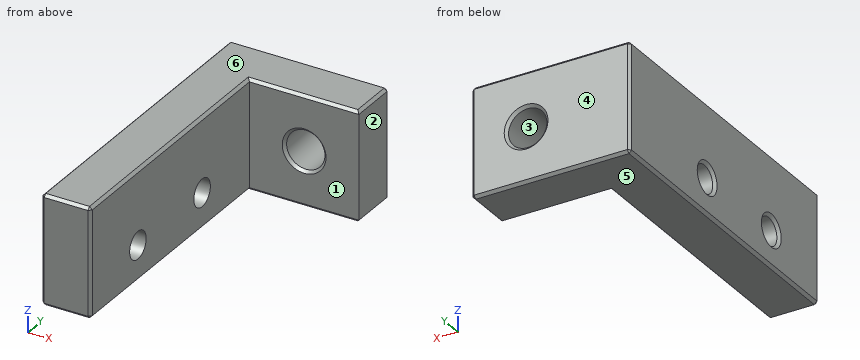
```python
from build123d import *

# Parameters (mm, degrees)
BOSS_EXTRUDE1_DEPTH = 10
SKETCH2_R           = 1.75
CUT_EXTRUDE1_DEPTH  = 10
SKETCH3_R           = 1.25
CUT_EXTRUDE2_DEPTH  = 10
CHAMFER1_SIZE       = 0.25


with BuildPart() as part:
    # Sketch1 → Boss-Extrude1 (new body)
    with BuildSketch(Plane.XY):
        Polygon((0, 0), (0, 28.5), (14.5, 28.5), (14.5, 24), (4.5, 24), (4.5, 0), align=None)
    extrude(amount=BOSS_EXTRUDE1_DEPTH)

    # Sketch2 → Cut-Extrude1 (cut)
    with BuildSketch(Plane.XZ.offset(-24)):
        with Locations((9.5, 5)):
            Circle(SKETCH2_R)
    extrude(amount=-CUT_EXTRUDE1_DEPTH, mode=Mode.SUBTRACT)

    # Sketch3 → Cut-Extrude2 (cut)
    with BuildSketch(Plane(origin=(4.5, 0, 0), x_dir=(0, 0, -1), z_dir=(1, 0, 0))):
        with Locations(Location((-3.25, 7.15, 0), (0, 0, 90))):
            Circle(SKETCH3_R)
        with Locations(Location((-3.25, 16.85, 0), (0, 0, 90))):
            Circle(SKETCH3_R)
    extrude(amount=-CUT_EXTRUDE2_DEPTH, mode=Mode.SUBTRACT)

    # Chamfer1
    chamfer1_edges = [part.edges().sort_by_distance(p)[0] for p in [
        (0, 0, 5),
        (0, 28.5, 5),
        (14.5, 28.5, 5),
        (4.5, 0, 5),
        (9.5, 24, 10),
        (14.5, 26.25, 10),
        (7.75, 28.5, 5),
        (7.25, 28.5, 10),
        (7.75, 24, 5),
        (0, 14.25, 10),
        (0, 5.9, 3.25),
        (0, 15.6, 3.25),
        (2.25, 0, 10),
        (0, 14.25, 0),
        (7.25, 28.5, 0),
        (14.5, 26.25, 0),
        (9.5, 24, 0),
        (4.5, 12, 0),
        (2.25, 0, 0),
        (4.5, 12, 10),
    ]]
    chamfer(chamfer1_edges, length=CHAMFER1_SIZE)


solid = part.part
```
Build history of the part. All positions in model axes, mm. Face numbers are marked on the shaded views. A direction names the side the tool comes from. Give positions to 0.01 mm unless a question says otherwise; leave off trailing zeros. Order: outer loops, then holes, each group sorted by start corner. A loop starts at its lowest first (then second) coordinate and runs counter-clockwise, first axis right, second up. Notation, with made-up numbers: M 34.25,43.5 L 92.25,43.5 A20 ccw 92.25,55.5 Z; hole C 66,55.25 d5. An arc over 180 degrees is marked long. Write item = value, one per line. Start each with the question number.
(1) Slice it at D-D on y = 4.5. Write the cut outline in (x, z).
(2) Two-plate mould, pull along Z, no slides. Class the marked faces 3, 4, 5 and 6: released by +Z, released by -Z, zero draft, split by the parting line, or undercut.
(3) Pin check, flat tips, straight feed: pin 1 Ø1 at (x, y) = (4.5, 18.5) entering from +Z; pin 2 Ø5 at (y, z) = (6.5, 5.5) entering from +X. Stop position of each tip, or through.
(4) Probe L1, parallel to Z at x = 9.5, y = 27.1; L2, parallel to Z at x = 3, y = 7.15; L3, parallel to Y at x = 4, z = 4. List the from-to ranges inside material, lowest first. Write a range as [from, to].
(5) Slice it at A-A on x = 9.5. Write the cut outline in (y, z).
(6) Slice it at C-C on z = 7.5. Write the cut outline in (x, y).
(7) Which spindle directions (+Z, -Z, +X, -X, +Y, -Y) get a long thin tool onto all of the face, cutting with end or side? Do the marked faces 1 and 2. Say none if no direction does.
(8) Slice it at B-B on y = 16.85. Write the cut outline in (x, z).
Responses:
q1.outline = M 0,0.25 L 0.25,0 L 4.25,0 L 4.5,0.25 L 4.5,9.75 L 4.25,10 L 0.25,10 L 0,9.75 Z
q2.face_3 = undercut
q2.face_4 = zero draft
q2.face_5 = released by -Z
q2.face_6 = released by +Z
q3.pin_1 = 10
q3.pin_2 = 4.5
q4.L1 = [0, 3.25], [6.75, 10]
q4.L2 = [0, 2], [4.5, 10]
q4.L3 = [0, 6.15], [8.15, 15.85], [17.85, 28.5]
q5.outline = M 24,0.25 L 24.25,0 L 28.25,0 L 28.5,0.25 L 28.5,3 L 28.25,3.25 L 24.25,3.25 L 24,3 Z; M 24,7 L 24.25,6.75 L 28.25,6.75 L 28.5,7 L 28.5,9.75 L 28.25,10 L 24.25,10 L 24,9.75 Z
q6.outline = M 0,0.25 L 0.25,0 L 4.25,0 L 4.5,0.25 L 4.5,24 L 14.5,24 L 14.5,28.25 L 14.25,28.5 L 0.25,28.5 L 0,28.25 Z
q7.face_1 = +Z, -Z, +X, -Y
q7.face_2 = +Z, -Z, +X, +Y, -Y
q8.outline = M 0,0.25 L 0.25,0 L 4.25,0 L 4.5,0.25 L 4.5,2 L 0.25,2 L 0,1.75 Z; M 0,4.75 L 0.25,4.5 L 4.5,4.5 L 4.5,9.75 L 4.25,10 L 0.25,10 L 0,9.75 Z
